from build123d import *

# Parameters (mm, degrees)
F0_R     = 19.0157086471
F1_DEPTH = 40.64
F0_R_2   = 10.5259508952
F2_DEPTH = 32.004
F3_W     = 16.7762897909
F3_H     = 49.2964833975
F4_DEPTH = 25.4


with BuildPart() as f1:
    # F0 (on Top) → F1 (new body)
    with BuildSketch(Plane.XY):
        with BuildLine():
            Line((25.8096773177, -32.5201936066), (25.8096773177, 16.7762897909))
            Line((25.8096773177, 16.7762897909), (-27.3582581431, 16.7762897909))
            ThreePointArc((-27.3582581431, 16.7762897909), (-52.0064998418, -7.8719519079), (-27.3582581431, -32.5201936066))
            Line((-27.3582581431, -32.5201936066), (25.8096773177, -32.5201936066))
        make_face()
        with Locations((-27.3582581431, -7.8719519079)):
            Circle(F0_R, mode=Mode.SUBTRACT)
    extrude(amount=F1_DEPTH)

    # F0 (on Top) → F2 (join)
    with BuildSketch(Plane.XY):
        with Locations((-27.3582581431, -7.8719519079)):
            Circle(F0_R)
        with Locations((-27.3582581431, -7.8719519079)):
            Circle(F0_R_2, mode=Mode.SUBTRACT)
    extrude(amount=F2_DEPTH)

    # F3 (on face) → F4 (cut)
    with BuildSketch(Plane.XY.offset(40.64)):
        with Locations((17.4215324223, -7.8719519079)):
            Rectangle(F3_W, F3_H)
    extrude(amount=-F4_DEPTH, mode=Mode.SUBTRACT)


solid = f1.part
CAD build for the part. Positions are in the model's coordinates, mm. A direction names the side the tool comes from. Coordinates: 2 decimals unless noted, no trailing zeros. Write each loop counter-clockwise with the first axis right and the second up, starting at its lowest first coordinate (ties: lowest second). Pieces come first, ordered by that corner, then holes. Notation, with made-up numbers: M 70,84.25 L 99,84.25 A25 cw 99,109.25 Z; hole C -38,31.25 d11. An arc over 180 degrees is marked long. Return JSON: item names as keys, results as strings.
Item 1: Which spindle directions (+Z, -Z, +X, -X, +Y, -Y) get a long thin tool onto all of the face, cutting with end or side? Do faces 1 (the cylindrical face through (-35.71, -14.28, 15.78)), 2 (the flat face through (9.033, -8, 28)), 3 (the cylindrical face through (-9.22, -2.16, 36.26)). Say none if no direction does.
Findings below:
{"face 1": "+Z, -Z", "face 2": "+Z, +X, +Y, -Y", "face 3": "+Z"}
Item 2: Probe line 1 (Z direction, x = 17, y = -27); line 2 (Y direction, x = -36.5, z = 19); line 3 (Z direction, x = -19.5, y = -18). List the from-to ranges inside material, lowest first. Write a range as from..to.
Findings below:
{"line 1": "z = 0..15.24", "line 2": "y = -30.76..-13.09, -2.65..15.02", "line 3": "z = 0..32"}
Item 3: Drop flat-ended pins along their axis: pin 1 Ø20.5 at (y, z) = (-2, 34.5) entering from +X; pin 2 Ø23 at (x, y) = (-27.36, -7.87) entering from +Z; pin 3 Ø5 at (x, y) = (17.5, -4) entering from +Z; pin 4 Ø24 at (x, y) = (-27.36, -7.87) entering from -Z. Give the stop position or say it passes through.
Findings below:
{"pin 1": "stops at x = 9.03", "pin 2": "stops at z = 32", "pin 3": "stops at z = 15.24", "pin 4": "stops at z = 0"}
Item 4: Two-plate mould, pull along Y, no slides. Class faces 4 (the flat face through (-19, -16, 32.004)), 5 (the flat face through (-7, -32.52, 20)), 6 (the cylindrical face through (-52, -7.3, 20)): +Y half, -Y half, draft (parallel to the pull), parting line (faces both ways), or undercut.
Findings below:
{"face 4": "undercut", "face 5": "-Y half", "face 6": "parting line"}
Item 5: Slice it at B-B, the plane y = -11. Write the cut outline in (x, z).
Findings below:
{"outline": "M -51.81,0 L -37.41,0 L -37.41,32 L -46.11,32 L -46.11,40.64 L -51.81,40.64 Z; M -17.31,0 L 25.81,0 L 25.81,15.24 L 9.03,15.24 L 9.03,40.64 L -8.6,40.64 L -8.6,32 L -17.31,32 Z"}
Item 6: Slice it at C-C, the plane z = 17. Write the cut outline in (x, y), and give its area (3 significant figures).
Findings below:
{"outline": "M -27.36,-32.52 L 9.03,-32.52 L 9.03,16.78 L -27.36,16.78 A24.65 ccw Z; hole C -27.36,-7.87 d21.05", "area": "2,400 mm2"}
Item 7: Slice it at D-D, the plane y = -26. Write the cut outline in (x, z).
Findings below:
{"outline": "M -44.06,0 L 25.81,0 L 25.81,15.24 L 9.03,15.24 L 9.03,40.64 L -21.62,40.64 L -21.62,32 L -33.1,32 L -33.1,40.64 L -44.06,40.64 Z"}
Item 8: Slice it at A-A, the plane x = -30. Write the cut outline in (y, z), and give its area (3 significant figures).
Findings below:
{"outline": "M -32.38,0 L -18.06,0 L -18.06,32 L -26.7,32 L -26.7,40.64 L -32.38,40.64 Z; M 2.32,0 L 16.63,0 L 16.63,40.64 L 10.96,40.64 L 10.96,32 L 2.32,32 Z", "area": "1,010 mm2"}
